```python
from build123d import *

# Parameters (mm, degrees)
SKETCH1_R           = 50
SKETCH1_R_2         = 13
SKETCH1_R_3         = 1.625
SKETCH1_R_4         = 2.65
BOSS_EXTRUDE1_DEPTH = 10
SKETCH2_R           = 3
CUT_EXTRUDE1_DEPTH  = 3
SKETCH3_R           = 4.375
CUT_EXTRUDE2_DEPTH  = 6
CHAMFER3_SIZE       = 1
CHAMFER4_SIZE       = 0.5


with BuildPart() as part:
    # Sketch1 → Boss-Extrude1 (new body)
    with BuildSketch(Plane(origin=(0, 0, 0), x_dir=(1, 0, 0), z_dir=(0, 1, 0))):
        with Locations(Location((0, 0, 0), (0, 0, 270))):
            Circle(SKETCH1_R)
        with Locations(Location((0, 0, 0), (0, 0, 270))):
            Circle(SKETCH1_R_2, mode=Mode.SUBTRACT)
        with Locations(Location((15.5, 15.5, 0), (0, 0, 270))):
            Circle(SKETCH1_R_3, mode=Mode.SUBTRACT)
        with Locations(Location((15.5, -15.5, 0), (0, 0, 270))):
            Circle(SKETCH1_R_3, mode=Mode.SUBTRACT)
        with Locations(Location((-15.5, -15.5, 0), (0, 0, 270))):
            Circle(SKETCH1_R_3, mode=Mode.SUBTRACT)
        with Locations(Location((-15.5, 15.5, 0), (0, 0, 270))):
            Circle(SKETCH1_R_3, mode=Mode.SUBTRACT)
        with Locations(Location((40.5, 0, 0), (0, 0, 270))):
            Circle(SKETCH1_R_4, mode=Mode.SUBTRACT)
        with Locations(Location((0, -40.5, 0), (0, 0, 270))):
            Circle(SKETCH1_R_4, mode=Mode.SUBTRACT)
        with Locations(Location((-40.5, 0, 0), (0, 0, 270))):
            Circle(SKETCH1_R_4, mode=Mode.SUBTRACT)
        with Locations(Location((0, 40.5, 0), (0, 0, 270))):
            Circle(SKETCH1_R_4, mode=Mode.SUBTRACT)
    extrude(amount=BOSS_EXTRUDE1_DEPTH)

    # Chamfer1: read off the stored shape, not the designer's step
    # Chamfer1 outline → Chamfer1 (revolve, cut)
    with BuildSketch(Plane.XY):
        Polygon((50, 10), (48, 10), (50, 8), align=None)
    revolve(axis=Axis((0, 0, 0), (0, 1, 0)), mode=Mode.SUBTRACT)

    # Sketch2 → Cut-Extrude1 (cut)
    with BuildSketch(Plane(origin=(0, 10, 0), x_dir=(1, 0, 0), z_dir=(0, 1, 0))):
        with Locations(Location((-15.5, 15.5, 0), (0, 0, 270))):
            Circle(SKETCH2_R)
        with Locations(Location((15.5, 15.5, 0), (0, 0, 270))):
            Circle(SKETCH2_R)
        with Locations(Location((15.5, -15.5, 0), (0, 0, 270))):
            Circle(SKETCH2_R)
        with Locations(Location((-15.5, -15.5, 0), (0, 0, 270))):
            Circle(SKETCH2_R)
    extrude(amount=-CUT_EXTRUDE1_DEPTH, mode=Mode.SUBTRACT)

    # Chamfer2: read off the stored shape, not the designer's step
    # Chamfer2 outline → Chamfer2 (revolve, cut)
    with BuildSketch(Plane.XY):
        Polygon((13, 10), (13, 9), (14, 10), align=None)
    revolve(axis=Axis((0, 0, 0), (0, 1, 0)), mode=Mode.SUBTRACT)

    # Sketch3 → Cut-Extrude2 (cut)
    with BuildSketch(Plane(origin=(0, 10, 0), x_dir=(1, 0, 0), z_dir=(0, 1, 0))):
        with Locations(Location((40.5, 0, 0), (0, 0, 270))):
            Circle(SKETCH3_R)
        with Locations(Location((0, -40.5, 0), (0, 0, 270))):
            Circle(SKETCH3_R)
        with Locations(Location((-40.5, 0, 0), (0, 0, 270))):
            Circle(SKETCH3_R)
        with Locations(Location((0, 40.5, 0), (0, 0, 270))):
            Circle(SKETCH3_R)
    extrude(amount=-CUT_EXTRUDE2_DEPTH, mode=Mode.SUBTRACT)

    # Chamfer3
    chamfer3_edges = [part.edges().sort_by_distance(p)[0] for p in [
        (40.5, 10, -4.375),
        (0, 10, 36.125),
        (-40.5, 10, -4.375),
        (0, 10, -44.875),
    ]]
    chamfer(chamfer3_edges, length=CHAMFER3_SIZE)

    # Chamfer4
    chamfer4_edges = [part.edges().sort_by_distance(p)[0] for p in [
        (-15.5, 10, 12.5),
        (15.5, 10, 12.5),
        (15.5, 10, -18.5),
        (-15.5, 10, -18.5),
    ]]
    chamfer(chamfer4_edges, length=CHAMFER4_SIZE)


solid = part.part
```
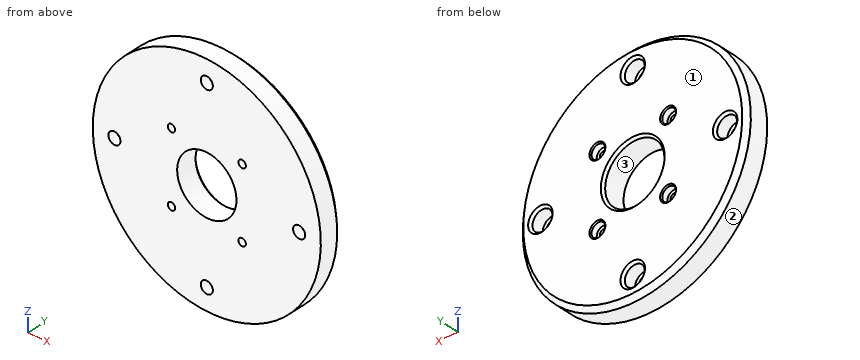
Verification items for the finished model (mm, model axes). Face numbers are marked on the shaded views. Round coordinates to 2 decimals unless told otherwise and drop trailing zeros. Answer as a JSON object with one key per item and string values. Group by question number.
Q1. Thickness scan on line 1 (X direction, y = 2.3, z = 0); line 2 (X direction, y = 6.45, z = 0) (3 decimals). Record the ranges inside material, lowest first.
Q2. Go/stop test with flat-tipped pins: pin 1 Ø1.9 at (x, z) = (-15.5, -15.5) entering from -Y; pin 2 Ø5 at (y, z) = (8, -4) entering from -X; pin 3 Ø1 at (x, y) = (16, 5) entering from -Z; pin 4 Ø3 at (x, z) = (-14.5, 14.5) entering from +Y. Record where each tip stops, or that it passes through.
Q3. Section check A-A, the plane z = 0. Give the number of separate pieces and of enclosed holes in the cut face, plus the area to 3 significant figures.
Q4. Mould release check, pull along X, two halves, no side actions. Record for the marked faces 1, 2 and 3: released by +X, released by -X, zero draft, split by the parting line, or undercut.
Found:
{
 "1": {"line 1": "x = -50 to -43.15, -37.85 to -13, 13 to 37.85, 43.15 to 50", "line 2": "x = -50 to -44.875, -36.125 to -13, 13 to 36.125, 44.875 to 50"},
 "2": {"pin 1": "passes through", "pin 2": "stops at x = -49.98", "pin 3": "stops at z = -47.54", "pin 4": "stops at y = 7"},
 "3": {"separate pieces": "4", "enclosed holes": "0", "area": "586 mm^2"},
 "4": {"face 1": "zero draft", "face 2": "split by the parting line", "face 3": "undercut"}
}
